from build123d import *

# Parameters (mm, degrees)
ESQUISSE1_W                                   = 15
ESQUISSE1_H                                   = 45
BOSS_EXTRU_1_DEPTH                            = 450
TROU_POUR_TARAUDAGE_POUR_TROU_TARAUD_M6_D     = 5
TROU_POUR_TARAUDAGE_POUR_TROU_TARAUD_M6_DEPTH = 10
TROU_POUR_TARAUDAGE_POUR_TROU_TARAUD_M6_TIP   = 1.502151548
TROU_POUR_TARAUDAGE_POUR_TROU_TARAUD_2_D      = 5
TROU_POUR_TARAUDAGE_POUR_TROU_TARAUD_2_DEPTH  = 10
TROU_POUR_TARAUDAGE_POUR_TROU_TARAUD_2_TIP    = 1.502151548
ESQUISSE10_W                                  = 20
ESQUISSE10_H                                  = 10
ENL_V_MAT_EXTRU_1_DEPTH                       = 15
TROU_POUR_TARAUDAGE_POUR_TROU_TARAUD_M5_D     = 4.2
TROU_POUR_TARAUDAGE_POUR_TROU_TARAUD_M5_DEPTH = 25
TROU_POUR_TARAUDAGE_POUR_TROU_TARAUD_M5_TIP   = 1.2618073


with BuildPart() as part:
    # Esquisse1 → Boss.-Extru.1 (new body)
    with BuildSketch(Plane.XY):
        with Locations((-7.5, 22.5)):
            Rectangle(ESQUISSE1_W, ESQUISSE1_H)
    extrude(amount=BOSS_EXTRU_1_DEPTH)

    # Trou pour taraudage pour trou taraud_ M6
    with Locations(Plane.XY.offset(450)):
        with Locations((-7.5, 35), (-7.5, 10)):
            Hole(TROU_POUR_TARAUDAGE_POUR_TROU_TARAUD_M6_D / 2, depth=TROU_POUR_TARAUDAGE_POUR_TROU_TARAUD_M6_DEPTH)
            with Locations((0, 0, -(TROU_POUR_TARAUDAGE_POUR_TROU_TARAUD_M6_DEPTH + TROU_POUR_TARAUDAGE_POUR_TROU_TARAUD_M6_TIP / 2))):  # 118° drill point
                Cone(0, TROU_POUR_TARAUDAGE_POUR_TROU_TARAUD_M6_D / 2, TROU_POUR_TARAUDAGE_POUR_TROU_TARAUD_M6_TIP, mode=Mode.SUBTRACT)

    # Trou pour taraudage pour trou taraud 2
    with Locations(Plane(origin=(0, 0, 0), x_dir=(-1, 0, 0), z_dir=(0, 0, -1))):
        with Locations((7.5, 35), (7.5, 10)):
            Hole(TROU_POUR_TARAUDAGE_POUR_TROU_TARAUD_2_D / 2, depth=TROU_POUR_TARAUDAGE_POUR_TROU_TARAUD_2_DEPTH)
            with Locations((0, 0, -(TROU_POUR_TARAUDAGE_POUR_TROU_TARAUD_2_DEPTH + TROU_POUR_TARAUDAGE_POUR_TROU_TARAUD_2_TIP / 2))):  # 118° drill point
                Cone(0, TROU_POUR_TARAUDAGE_POUR_TROU_TARAUD_2_D / 2, TROU_POUR_TARAUDAGE_POUR_TROU_TARAUD_2_TIP, mode=Mode.SUBTRACT)

    # Esquisse10 → Enlèv. mat.-Extru.1 (cut)
    with BuildSketch(Plane(origin=(0, 0, 0), x_dir=(0, 0, -1), z_dir=(1, 0, 0))):
        with Locations((-225, 40)):
            Rectangle(ESQUISSE10_W, ESQUISSE10_H)
    extrude(amount=-ENL_V_MAT_EXTRU_1_DEPTH, mode=Mode.SUBTRACT)

    # Trou pour taraudage pour trou taraudé M51
    with Locations(Plane(origin=(0, 45, 0), x_dir=(1, 0, 0), z_dir=(0, 1, 0))):
        with Locations((-7.5, -430), (-7.5, -255), (-7.5, -195), (-7.5, -20)):
            Hole(TROU_POUR_TARAUDAGE_POUR_TROU_TARAUD_M5_D / 2, depth=TROU_POUR_TARAUDAGE_POUR_TROU_TARAUD_M5_DEPTH)
            with Locations((0, 0, -(TROU_POUR_TARAUDAGE_POUR_TROU_TARAUD_M5_DEPTH + TROU_POUR_TARAUDAGE_POUR_TROU_TARAUD_M5_TIP / 2))):  # 118° drill point
                Cone(0, TROU_POUR_TARAUDAGE_POUR_TROU_TARAUD_M5_D / 2, TROU_POUR_TARAUDAGE_POUR_TROU_TARAUD_M5_TIP, mode=Mode.SUBTRACT)


solid = part.part
For this review, take the finished solid that the model builds, in its own axes (mm). A direction names the side the tool comes from. Round coordinates to 2 decimals unless told otherwise and drop trailing zeros. Order: outer loops, then holes, each group sorted by start corner. A loop starts at its lowest first (then second) coordinate and runs counter-clockwise, first axis right, second up. Notation, with made-up numbers: (54, -18) -> (113, -18) arc R19 cw to (113, -13) -> close; hole circle Ø5 at (-25, 29). An arc over 180 degrees is marked (long way). Put each result on its own line as item: value.
Q1. Mouldability with a two-part tool opening along Z and no side actions: class faces 3 (the flat face through (-7, 40, 215)), 4 (the flat face through (-8, 23, 0)), 5 (the flat face through (-8, 45, 341)) as pulls with the +Z half, pulls with the -Z half, needs draft (parallel to the pull), parting line crosses it, or undercut.
Check result:
face 3: undercut
face 4: pulls with the -Z half
face 5: needs draft
Q2. For probe 1 along Z at (x, y) = (-7.5, 38.75); probe 2 along Z at (x, y) = (-7.5, 27.5); probe 3 along Y at (x, z) = (-7.5, 6), list the stretches that pass through material, from the lowest coordinate up. Write a range as [from, to].
Check result:
probe 1: [0, 17.9], [22.1, 192.9], [197.1, 215], [235, 252.9], [257.1, 427.9], [432.1, 450]
probe 2: [0, 17.9], [22.1, 192.9], [197.1, 252.9], [257.1, 427.9], [432.1, 450]
probe 3: [0, 7.5], [12.5, 32.5], [37.5, 45]
Q3. Add section A-A on z = 220. Write out the cut boundary in (x, y), plus the area to 3 significant figures.
Check result:
outline: (-15, 0) -> (0, 0) -> (0, 35) -> (-15, 35) -> close
area: 525 mm2
Q4. Machinability: for faces 1 (the flat face through (-7, 40, 235)), 2 (the flat face through (-8, 0, 222)), which of the approach directions +Z, -Z, +X, -X, +Y, -Y give a long, thin tool a straight path to every point of the face, cutting with its end or side? Answer none if there is none.
Check result:
face 1: +X, -X, +Y
face 2: +Z, -Z, +X, -X, -Y
Q5. Insertion check: pin 1 Ø2.5 at (x, z) = (-7.5, 255) entering from +Y; pin 2 Ø7.5 at (x, z) = (-6, 229) entering from +Y; pin 3 Ø4 at (x, y) = (-7.5, 35) entering from -Z. Each pin has a flat end and moves straight along its axis. Give the tip position at first contact, or say it passes through.
Check result:
pin 1: y = 19.49
pin 2: y = 35
pin 3: z = 10.3
